```python
from build123d import *

# Parameters (mm, degrees)
BOSS_EXTRUDE1_DEPTH     = 25
CUT_EXTRUDE1_DEPTH      = 26.350366738
CUT_EXTRUDE1_DEPTH_BACK = 26.350366738
CHAMFER1_SIZE           = 0.5


with BuildPart() as part:
    # Sketch1 → Boss-Extrude1 (new body)
    with BuildSketch(Plane(origin=(0, 0, 0), x_dir=(1, 0, 0), z_dir=(0, 1, 0))):
        Polygon((0, 3.175), (-2.749630657, 1.5875), (-2.749630657, -1.5875), (0, -3.175), (2.749630657, -1.5875), (2.749630657, 1.5875), align=None)
    extrude(amount=BOSS_EXTRUDE1_DEPTH)

    # Sketch2 → Cut-Extrude1 (cut, two sides: drawn at the far end of the back side and taken through both)
    with BuildSketch(Plane.XY.offset(-CUT_EXTRUDE1_DEPTH_BACK)):
        with BuildLine():
            Line((-2.749630657, 25), (-0.5, 25))
            ThreePointArc((-0.5, 25), (-0.978721639, 19.854652783), (-2.749630657, 15))
            Line((-2.749630657, 15), (-2.749630657, 25))
        make_face()
        with BuildLine():
            Line((0.5, 25), (2.749630657, 25))
            Line((2.749630657, 25), (2.749630657, 15))
            ThreePointArc((2.749630657, 15), (0.978721639, 19.854652783), (0.5, 25))
        make_face()
    extrude(amount=CUT_EXTRUDE1_DEPTH + CUT_EXTRUDE1_DEPTH_BACK, mode=Mode.SUBTRACT)

    # Chamfer1
    chamfer1_edges = [part.edges().sort_by_distance(p)[0] for p in [
        (2.749630657, 0, 0),
        (1.374815329, 0, 2.38125),
        (-1.374815329, 0, 2.38125),
        (-2.749630657, 0, 0),
        (-1.374815329, 0, -2.38125),
        (1.374815329, 0, -2.38125),
    ]]
    chamfer(chamfer1_edges, length=CHAMFER1_SIZE)


solid = part.part
```
Input: part model. Units: mm. Frame: model coordinates. Give positions to 0.01 mm unless a question says otherwise; leave off trailing zeros. Loops run counter-clockwise (first coordinate to the right, second up) from the corner with the lowest first, then second, coordinate; pieces in that order, holes last.
1) Section query C-C on x = 1.7. Return the cut outline in (y, z).
A:
outline: (0, -1.62) - (0.5, -2.19) - (17.39, -2.19) - (17.39, 2.19) - (0.5, 2.19) - (0, 1.62) - close
2) Section query A-A on z = 0. Return the cut outline in (x, y), and give its area (3 significant figures).
A:
outline: (-2.75, 0.5) - (-2.25, 0) - (2.25, 0) - (2.75, 0.5) - (2.75, 15) arc R20.16 cw to (0.5, 25) - (-0.5, 25) arc R20.16 cw to (-2.75, 15) - close
area: 106 mm2
3) Section query B-B on y = 20.5. Return the cut outline in (x, z) (3 decimals).
A:
outline: (-0.845, -2.687) - (0, -3.175) - (0.845, -2.687) - (0.845, 2.687) - (0, 3.175) - (-0.845, 2.687) - close
4) Line query: L1, parallel to Z at x = 1.25, y = 1; L2, parallel to Z at x = -1.05, y = 15; L3, parallel to Y at x = -2.3, z = -1.75. Output: solid intervals per line, ascending.
A:
L1: z = -2.45 to 2.45
L2: z = -2.57 to 2.57
L3: y = 0.42 to 15.92
